Geometry check sheet. Reference: the model listing, model coordinates, mm. Face numbers are marked on the shaded views. Coordinates: 2 decimals unless noted, no trailing zeros. Write each loop counter-clockwise with the first axis right and the second up, starting at its lowest first coordinate (ties: lowest second). Pieces come first, ordered by that corner, then holes. Notation, with made-up numbers: (-23.75, -2) -> (5.25, -2) arc R25 ccw to (5.25, 29) -> close; hole circle Ø6 at (27.25, -1). An arc over 180 degrees is marked (long way). One line per question, with ' | ' between items.
from build123d import *

# Parameters (mm, degrees)
SKETCH_1_R      = 11.25
SKETCH_1_R_2    = 1.5
EXTRUDE_1_DEPTH = 5


with BuildPart() as part:
    # 草图1 → 凸台-拉伸1 (new body)
    with BuildSketch(Plane(origin=(0, 0, 0), x_dir=(1, 0, 0), z_dir=(0, 1, 0))):
        Polygon((-34.5, 21.15), (34.5, 21.15), (34.5, 16.15), (39.5, 16.15), (39.5, 6.15), (34.5, 6.15), (34.5, -6.15), (39.5, -6.15), (39.5, -16.15), (34.5, -16.15), (34.5, -21.15), (24.5, -21.15), (24.5, -26.15), (14.5, -26.15), (14.5, -21.15), (-14.5, -21.15), (-14.5, -26.15), (-24.5, -26.15), (-24.5, -21.15), (-34.5, -21.15), (-34.5, -16.15), (-39.5, -16.15), (-39.5, -6.15), (-34.5, -6.15), (-34.5, 6.15), (-39.5, 6.15), (-39.5, 16.15), (-34.5, 16.15), align=None)
        with Locations(Location((10.5, 0, 0), (0, 0, 270))):
            Circle(SKETCH_1_R, mode=Mode.SUBTRACT)
        with Locations(Location((-6.134831461, 16.634831461, 0), (0, 0, 270))):
            Circle(SKETCH_1_R_2, mode=Mode.SUBTRACT)
        with Locations(Location((27.134831461, 16.634831461, 0), (0, 0, 270))):
            Circle(SKETCH_1_R_2, mode=Mode.SUBTRACT)
        with Locations(Location((-6.134831461, -16.634831461, 0), (0, 0, 270))):
            Circle(SKETCH_1_R_2, mode=Mode.SUBTRACT)
        with Locations(Location((27.134831461, -16.634831461, 0), (0, 0, 270))):
            Circle(SKETCH_1_R_2, mode=Mode.SUBTRACT)
    extrude(amount=EXTRUDE_1_DEPTH)


solid = part.part
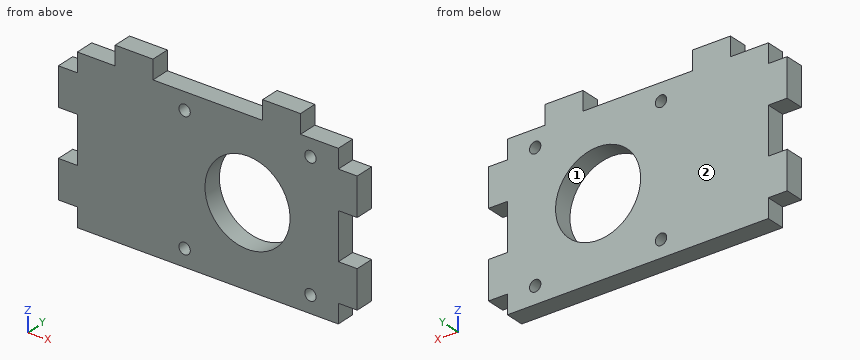
1. Cross-section at B-B on x = 10.5. Record the boundary of the cut face in (y, z).
Worked answers:
outline: (0, -21.15) -> (5, -21.15) -> (5, -11.25) -> (0, -11.25) -> close; (0, 11.25) -> (5, 11.25) -> (5, 21.15) -> (0, 21.15) -> close
2. Go/stop test with flat-tipped pins: P1, Ø2.5, axis at x = 37.5, y = 3.5, coming from the +Z side; P2, Ø2.5, axis at x = -6.13, z = -16.63, coming from the +Y side; P3, Ø2.5, axis at y = 3.5, z = 19, coming from the +X side; P4, Ø1.5, axis at x = -29, y = 3, coming from the +Z side. Record where each tip stops, or that it passes through.
Worked answers:
P1: z = 16.15 | P2: through | P3: x = 34.5 | P4: z = 21.15
3. Cross-section at D-D on x = 30.5. Record the boundary of the cut face in (y, z), and give its area (4 significant figures).
Worked answers:
outline: (0, -21.15) -> (5, -21.15) -> (5, 21.15) -> (0, 21.15) -> close | area: 211.5 mm²
4. Cross-section at A-A on z = 9. Record the boundary of the cut face in (x, y).
Worked answers:
outline: (-39.5, 0) -> (3.75, 0) -> (3.75, 5) -> (-39.5, 5) -> close; (17.25, 0) -> (39.5, 0) -> (39.5, 5) -> (17.25, 5) -> close
5. Mould release check, pull along X, two halves, no side actions. Record for the marked faces 1 and 2: released by +X, released by -X, zero draft, split by the parting line, or undercut.
Worked answers:
face 1: undercut | face 2: zero draft
6. Cross-section at C-C on y = 0.9. Give the number of separate pieces and of enclosed holes in the cut face, and give its area (3 significant figures).
Worked answers:
separate pieces: 1 | enclosed holes: 5 | area: 2,790 mm²
7. Material ranges on line 1 (Z direction, x = 35.5, y = 2.75); line 2 (X direction, y = 3.05, z = 0); line 3 (X direction, y = 2.1, z = 17), recorded low to high. Write a range as from..to.
Worked answers:
line 1: -16.15..-6.15, 6.15..16.15 | line 2: -34.5..-0.75, 21.75..34.5 | line 3: -34.5..-7.59, -4.68..25.68, 28.59..34.5
